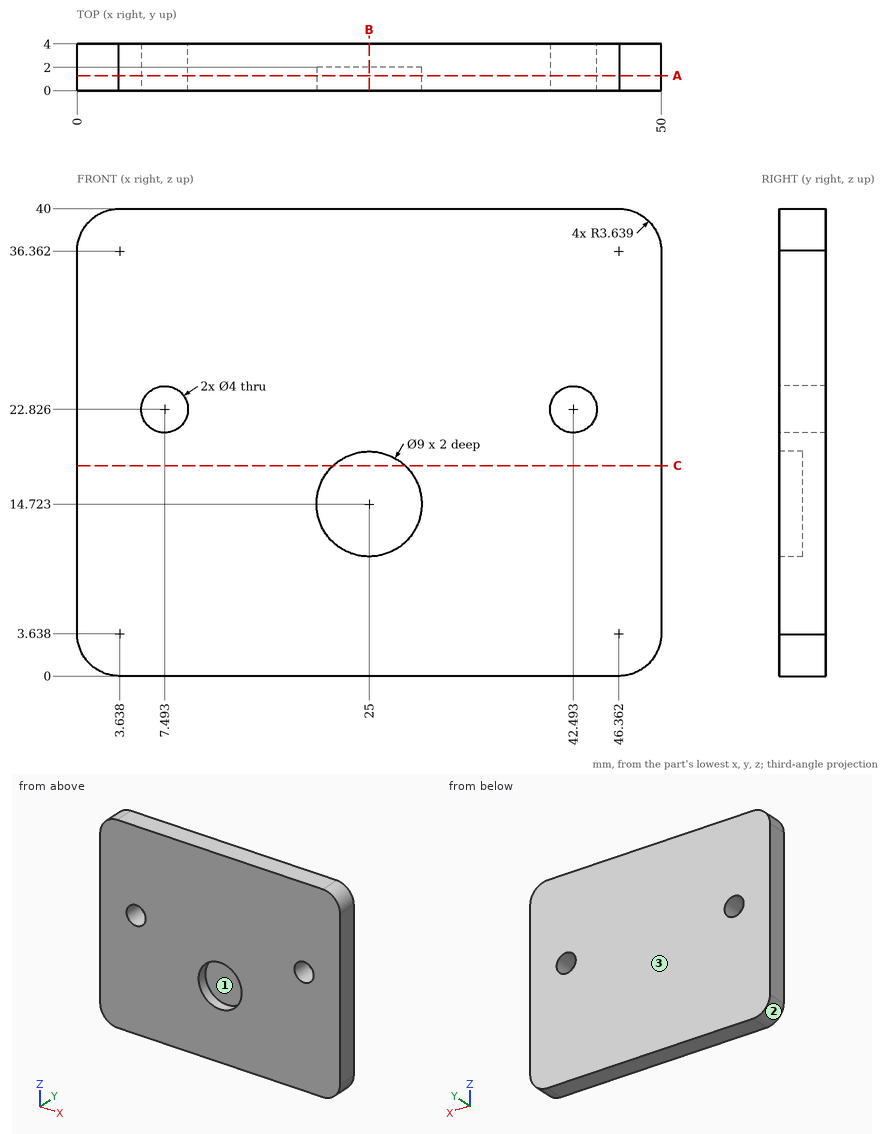
Here's the drawing with two shaded views (mm, measured from the low corner). I have some questions. Round coordinates to 2 decimals unless told otherwise and drop trailing zeros. Order: outer loops, then holes, each group sorted by start corner. A loop starts at its lowest first (then second) coordinate and runs counter-clockwise, first axis right, second up. Notation, with made-up numbers: (64, 17) -> (123, 17) arc R19 cw to (123, 24) -> close; hole circle Ø10 at (18.5, 56.5). An arc over 180 degrees is marked (long way). Write each question's results on one line, items separated by ' | '. Start each with the question number.
Item 1: If we section it at C-C, the plane z = 18: Write out the boundary of the cut face in (x, y) (1 decimal), then the cut area to 3 significant figures.
Item 2: If we section it at B-B, the plane x = 25: Write out the boundary of the cut face in (y, z).
Item 3: Will this pin go through, and if not, where does the flat tip stop? pin 1 (4.5 mm diameter, centred on x = 25, z = 14.5, fed in from -Y).
Item 4: If we section it at A-A, the plane y = 1.3: Write out the boundary of the cut face in (x, z).
Item 5: Please list where these lines run through material, in increasing order: L1, parallel to X at y = 1.3, z = 15; L2, parallel to Z at x = 25, y = 1.45; L3, parallel to X at y = 0.75, z = 21.5 (1 decimal).
Item 6: Thinking about a two-plate mould opening in X: for the marked faces 1, 2 and 3, which applies, +X half, -X half, draft (parallel to the pull), parting line (faces both ways), or undercut?
Results:
1) outline: (0, 0) -> (21.9, 0) -> (21.9, 2) -> (28.1, 2) -> (28.1, 0) -> (50, 0) -> (50, 4) -> (0, 4) -> close | area: 188 mm2
2) outline: (0, 0) -> (4, 0) -> (4, 40) -> (0, 40) -> (0, 19.22) -> (2, 19.22) -> (2, 10.22) -> (0, 10.22) -> close
3) pin 1: stops at y = 2
4) outline: (0, 3.55) arc R3.64 ccw to (3.55, 0) -> (46.45, 0) arc R3.64 ccw to (50, 3.55) -> (50, 36.45) arc R3.64 ccw to (46.45, 40) -> (3.55, 40) arc R3.64 ccw to (0, 36.45) -> close; hole circle Ø4 at (7.49, 22.83); hole circle Ø9 at (25, 14.72); hole circle Ø4 at (42.49, 22.83)
5) L1: x = 0 to 20.51, 29.49 to 50 | L2: z = 0 to 10.22, 19.22 to 40 | L3: x = 0 to 6, 9 to 41, 44 to 50
6) face 1: undercut | face 2: -X half | face 3: draft
